Verification items for the finished model (mm, model axes). A direction names the side the tool comes from. Coordinates: 2 decimals unless noted, no trailing zeros. Write each loop counter-clockwise with the first axis right and the second up, starting at its lowest first coordinate (ties: lowest second). Pieces come first, ordered by that corner, then holes. Notation, with made-up numbers: (77.25, 14) -> (82.25, 14) arc R9 ccw to (82.25, 21) -> close; hole circle Ø1 at (34, 58). An arc over 180 degrees is marked (long way). Use a Markdown table: item, result. Add a question column.
from build123d import *

# Parameters (mm, degrees)
CUT_EXTRUDE_1_DEPTH = 16
CUT_EXTRUDE_2_DEPTH = 2.5
FILLET_1_R          = 1
CHAMFER_1_SIZE      = 0.5


with BuildPart() as part:
    # 草图2 → 旋转1 (revolve)
    with BuildSketch(Plane.XY, mode=Mode.PRIVATE) as revolve_1_sk:
        Polygon((-89.5, 0), (-89.5, 7.5), (-71.5, 7.5), (-71.5, 9), (-39.5, 9), (-39.5, 12.5), (-31, 12.5), (-31, 15.5), (-24, 15.5), (-24, 12.5), (0, 12.5), (0, 9), (16, 9), (16, 0), align=None)
    revolve(revolve_1_sk.sketch.rotate(Axis((-90.878838174, 0, 0), (1, 0, 0)), 90), axis=Axis((-90.878838174, 0, 0), (1, 0, 0)))

    # 草图3 → 切除-拉伸1 (cut)
    with BuildSketch(Plane(origin=(16, 0, 0), x_dir=(0, 0, -1), z_dir=(1, 0, 0))):
        with BuildLine():
            ThreePointArc((-2.741378302, 8.572330197), (-6.363961031, 6.363961031), (-8.572330197, 2.741378302))
            Line((-8.572330197, 2.741378302), (-2.741378302, 8.572330197))
        make_face()
        with BuildLine():
            Line((-2.741378302, -8.572330197), (-8.572330197, -2.741378302))
            ThreePointArc((-8.572330197, -2.741378302), (-6.363961031, -6.363961031), (-2.741378302, -8.572330197))
        make_face()
        with BuildLine():
            Line((8.572330197, -2.741378302), (2.741378302, -8.572330197))
            ThreePointArc((2.741378302, -8.572330197), (6.363961031, -6.363961031), (8.572330197, -2.741378302))
        make_face()
        with BuildLine():
            ThreePointArc((8.572330197, 2.741378302), (6.363961031, 6.363961031), (2.741378302, 8.572330197))
            Line((2.741378302, 8.572330197), (8.572330197, 2.741378302))
        make_face()
    extrude(amount=-CUT_EXTRUDE_1_DEPTH, mode=Mode.SUBTRACT)

    # 草图5 → 切除-拉伸2 (cut)
    with BuildSketch(Plane.XY.offset(9)):
        with BuildLine():
            Line((-64.5, 3), (-48.5, 3))
            ThreePointArc((-48.5, 3), (-45.5, 0), (-48.5, -3))
            Line((-48.5, -3), (-64.5, -3))
            ThreePointArc((-64.5, -3), (-67.5, 0), (-64.5, 3))
        make_face()
    extrude(amount=-CUT_EXTRUDE_2_DEPTH, mode=Mode.SUBTRACT)

    # 圆角1
    fillet_1_edges = [part.edges().sort_by_distance(p)[0] for p in [
        (16, -9, 0),
        (16, 0, -9),
        (16, 9, 0),
        (16, 0, 9),
    ]]
    fillet(fillet_1_edges, radius=FILLET_1_R - 0.0001)  # a hair under: the kernel refuses the full size

    # 倒角1
    chamfer_1_edges = [part.edges().sort_by_distance(p)[0] for p in [
        (0, 0, -12.5),
        (-24, 0, -15.5),
        (-31, 0, -15.5),
        (-39.5, 0, -12.5),
        (-71.5, 0, -7.5),
        (-89.5, 0, -7.5),
    ]]
    chamfer(chamfer_1_edges, length=CHAMFER_1_SIZE)


solid = part.part
1) Release check for a two-part mould opening along Y. For faces 4 (the face through (8.112, 5.616, 5.698)), 5 (the face through (8, 0, 9)), 6 (the face through (-56, 0, 6.5)) record: released by +Y, released by -Y, zero draft, split by the parting line, or undercut.
2) Gauge pin test, flat ends, axial feed: pin 1 (0.6 mm diameter, centred on x = -60, z = 7.5, fed in from +Y); pin 2 (1 mm diameter, centred on x = -55, z = 7, fed in from -Y); pin 3 (2 mm diameter, centred on x = -54, z = 4, fed in from -Y); pin 4 (1 mm diameter, centred on x = -58, z = 10, fed in from +Y). Record the tip position at first contact, or that the pin passes through.
3) Thickness scan on L1, parallel to Z at x = 4, y = 0; L2, parallel to X at y = -7, z = -12; L3, parallel to X at y = 6.5, z = 5.5. Record the ranges inside material, lowest first.
4) Set-up check for faces 1 (the face through (8.112, 5.698, -5.616)), 2 (the face through (-34.944, -3.755, 11.923)), 3 (the face through (-12.086, -3.755, 11.923)): record each of +Z, -Z, +X, -X, +Y, -Y from which the full face is reachable in a straight line by a thin tool's end or side.
5) Cross-section at A-A on x = -38. Record the boundary of the cut face in (y, z).
Returned:
| question | item | result |
|---|---|---|
| 1 | face 4 | released by +Y |
| 1 | face 5 | split by the parting line |
| 1 | face 6 | undercut |
| 2 | pin 1 | stops at y = 5.4 |
| 2 | pin 2 | stops at y = -6.22 |
| 2 | pin 3 | stops at y = -8.49 |
| 2 | pin 4 | passes through |
| 3 | L1 | z = -9 to 9 |
| 3 | L2 | x = -31 to -24 |
| 3 | L3 | x = -71.5 to 0 |
| 4 | face 1 | -Z, +X, +Y |
| 4 | face 2 | -X |
| 4 | face 3 | +X |
| 5 | outline | circle Ø25 at (0, 0) |
